```python
from build123d import *

# Parameters (mm, degrees)
EXTRUDE_4_DEPTH     = 15
SKETCH_4_R          = 15
EXTRUDE_5_DEPTH     = 17
SKETCH_6_R          = 10.1
CUT_EXTRUDE_1_DEPTH = 2


with BuildPart() as part:
    # ｽｹｯﾁ2 → ﾎﾞｽ - 押し出し4 (new body)
    with BuildSketch(Plane(origin=(0, 0, 0), x_dir=(1, 0, 0), z_dir=(0, 1, 0))):
        with BuildLine():
            ThreePointArc((-53.82643789, -36.437818048), (-56.846261527, -34.367935813), (-60.466933112, -34.910600109))
            Line((-60.466933112, -34.910600109), (-64.807406984, -37.416573868))
            ThreePointArc((-64.807406984, -37.416573868), (-67.177509772, -40.614402853), (-66.461234116, -44.529814279))
            ThreePointArc((-66.461234116, -44.529814279), (49.665387485, -62.716419588), (58.57572973, 54.487465409))
            Line((58.57572973, 54.487465409), (57.289371136, 55.838409315))
            Line((57.289371136, 55.838409315), (25.911523347, 88.791671712))
            ThreePointArc((25.911523347, 88.791671712), (19.306695871, 93.382511176), (11.427401304, 95))
            Line((11.427401304, 95), (0, 95))
            ThreePointArc((0, 95), (-15, 80), (0, 65))
            ThreePointArc((0, 65), (57.41714976, -30.467538684), (-53.82643789, -36.437818048))
        make_face()
    extrude(amount=EXTRUDE_4_DEPTH)

    # ｽｹｯﾁ4 → ﾎﾞｽ - 押し出し5 (add)
    with BuildSketch(Plane(origin=(0, 15, 0), x_dir=(1, 0, 0), z_dir=(0, 1, 0))):
        with Locations(Location((0, 80, 0), (0, 0, 270))):
            Circle(SKETCH_4_R)
    extrude(amount=EXTRUDE_5_DEPTH)

    # ｽｹｯﾁ6 → ｶｯﾄ - 押し出し1 (cut)
    with BuildSketch(Plane(origin=(0, 32, 0), x_dir=(1, 0, 0), z_dir=(0, 1, 0))):
        with Locations(Location((0, 80, 0), (0, 0, 270))):
            Circle(SKETCH_6_R)
    extrude(amount=-CUT_EXTRUDE_1_DEPTH, mode=Mode.SUBTRACT)


solid = part.part
```
Verification items for the finished model (mm, model axes). A direction names the side the tool comes from. Round coordinates to 2 decimals unless told otherwise and drop trailing zeros. Write each loop counter-clockwise with the first axis right and the second up, starting at its lowest first coordinate (ties: lowest second). Pieces come first, ordered by that corner, then holes. Notation, with made-up numbers: (42.25, 13) -> (57.25, 13) arc R15 cw to (57.25, 17) -> close; hole circle Ø5 at (-38, 52.25). An arc over 180 degrees is marked (long way). Write each question's results on one line, items separated by ' | '. Start each with the question number.
1. Draft check along X on faces 1 (the cylindrical face through (-14.967, 12.22, -80.989)), 2 (the flat face through (6, 7, -95)), 3 (the cylindrical face through (58.27, 7.4, 28.8)). Enter one of: +X half, -X half, draft (parallel to the pull), parting line (faces both ways), or undercut.
2. Cross-section at D-D (x = -44.5). Enter the section's corners in (y, z), then the cut area to 3 significant figures.
3. Cross-section at B-B (x = 40.5). Enter the section's corners in (y, z).
4. Material ranges on probe 1 along X at (y, z) = (30.75, -80); probe 2 along Z at (x, y) = (0, 7.75); probe 3 along Y at (x, z) = (61.5, 22), recorded low to high. Write a range as from..to.
5. Cross-section at C-C (z = 0). Enter the section's corners in (x, y), then the cut area to 3 significant figures.
6. Cross-section at A-A (y = 5.5). Enter the section's corners in (x, z).
7. Set-up check for faces 4 (the flat face through (66, 0, 5)), 5 (the flat face through (0, 30, -80)): record each of +Z, -Z, +X, -X, +Y, -Y from which the full face is reachable in a straight line by a thin tool's end or side.
8. Depth check by flat-ended pin: P1, Ø8, axis at y = 11.5, z = -45, coming from the -X side; P2, Ø6, axis at x = -43.5, y = 17.5, coming from the +Z side; P3, Ø10, axis at x = -2.5, z = -79, coming from the +Y side. Enter the tip coordinate at first touch or a pass-through.
Solutions:
1) face 1: parting line | face 2: draft | face 3: undercut
2) outline: (0, 47.38) -> (15, 47.38) -> (15, 66.48) -> (0, 66.48) -> close | area: 287 mm2
3) outline: (0, -73.47) -> (15, -73.47) -> (15, -50.84) -> (0, -50.84) -> close; (0, 50.84) -> (15, 50.84) -> (15, 68.99) -> (0, 68.99) -> close
4) probe 1: x = -15..-10.1, 10.1..15 | probe 2: z = -95..-65, 65..80 | probe 3: y = 0..15
5) outline: (65, 0) -> (80, 0) -> (80, 15) -> (65, 15) -> close | area: 225 mm2
6) outline: (-66.46, 44.53) arc R5 ccw to (-64.81, 37.42) -> (-60.47, 34.91) arc R5 ccw to (-53.83, 36.44) arc R65 cw (long way) to (0, -65) arc R15 ccw to (0, -95) -> (11.43, -95) arc R20 ccw to (25.91, -88.79) -> (58.58, -54.49) arc R80 ccw (long way) to start
7) face 4: +Z, -Z, +X, -X, -Y | face 5: +Y
8) P1: stops at x = 42.71 | P2: stops at z = 68.19 | P3: stops at y = 30
